Autodesk Inventor part; units mm, degrees
ref_plane "YZ Plane" through (0, 0, 0) normal (1, 0, 0) x (0, 1, 0)
ref_plane "XZ Plane" through (0, 0, 0) normal (0, 1, 0) x (-1, 0, 0)
ref_plane "XY Plane" through (0, 0, 0) normal (0, 0, 1) x (1, 0, 0)
sketch "Sketch6" plane through (0, 0, 0) normal (0, 1, 0) x (-1, 0, 0)
  line L0 (306.3, -490) -> (-306.3, -490)
  line L1 (-306.3, -490) -> (-306.3, 490)
  line L2 (-306.3, 490) -> (306.3, 490)
  line L3 (306.3, 490) -> (306.3, -490)
  line L4 (306.3, -490) -> (-306.3, 490) construction
  line L5 (-306.3, -490) -> (306.3, 490) construction
  point P0 (0, 0)
  dimension "d52" = 612.6
  dimension "d53" = 980
extrude "Plate2" add sketch "Sketch6" along normal blind 0.5
sketch "Sketch11" plane through (-305.8, 0, 490) normal (-1, 0, 0) x (0, -1, 0)
  line L0 (0, -980) -> (0, 0)
  line L1 (0, 0) -> (-10, 0)
  line L2 (-10, 0) -> (-10, -980)
  line L3 (-10, -980) -> (0, -980)
edge flange "Flange2" height 10 angle 90 thickness 0.5 bend radius 0.5 thickness toward (-1, 0, 0) relief tear relief width 0.5 relief depth 0.25 edges at (-306.3, 0.5, 0) wall of the first edge with corners at (-305.8, 0, -490) (-305.8, 0, 490) (-305.8, 10, 490) (-305.8, 10, -490)
bend "Bend3"
corner "Corner3"
sketch "Sketch12" plane through (-306.3, 9.5, 490) normal (0, 1, 0) x (-1, 0, 0)
  line L0 (0, -980) -> (0, 0)
  line L1 (0, 0) -> (-10, 0)
  line L2 (-10, 0) -> (-10, -980)
  line L3 (-10, -980) -> (0, -980)
edge flange "Flange3" height 10 angle 90 thickness 0.5 bend radius 0.5 thickness toward (0, 1, 0) relief tear relief width 0.5 relief depth 0.25 edges at (-305.8, 10, 0) wall of the first edge with corners at (-306.3, 9.5, -490) (-306.3, 9.5, 490) (-296.3, 9.5, 490) (-296.3, 9.5, -490)
bend "Bend4"
corner "Corner4"
sketch "Sketch13" plane through (305.8, 0, -490) normal (1, 0, 0) x (0, 1, 0)
  line L0 (0, 980) -> (0, 0)
  line L1 (0, 0) -> (10, 0)
  line L2 (10, 0) -> (10, 980)
  line L3 (10, 980) -> (0, 980)
edge flange "Flange4" height 10 angle 90 thickness 0.5 bend radius 0.5 thickness toward (1, 0, 0) relief tear relief width 0.5 relief depth 0.25 edges at (306.3, 0.5, 0) wall of the first edge with corners at (305.8, 0, 490) (305.8, 0, -490) (305.8, 10, -490) (305.8, 10, 490)
bend "Bend5"
corner "Corner5"
sketch "Sketch14" plane through (306.3, 9.5, -490) normal (0, 1, 0) x (-1, 0, 0)
  line L0 (0, 980) -> (0, 0)
  line L1 (0, 0) -> (10, 0)
  line L2 (10, 0) -> (10, 980)
  line L3 (10, 980) -> (0, 980)
edge flange "Flange5" height 10 angle 90 thickness 0.5 bend radius 0.5 thickness toward (0, 1, 0) relief tear relief width 0.5 relief depth 0.25 edges at (305.8, 10, 0) wall of the first edge with corners at (306.3, 9.5, 490) (306.3, 9.5, -490) (296.3, 9.5, -490) (296.3, 9.5, 490)
bend "Bend6"
corner "Corner6"
fillet "Corner Round1" radius 4 4 edges at (296.3, 9.75, -490) (296.3, 9.75, 490) (-296.3, 9.75, -490) (-296.3, 9.75, 490)
equation "\"d52\" = ЖАБРЫ_базовая_ширина - 3 * ЖАБРЫ_шаг_листов"
equation "\"d53\" = ЖАБРЫ_базовая_длина_кор_лист"
equation "\"d54\" = Thickness"
equation "\"d84\" = BendReliefWidth"
equation "\"d85\" = BendReliefDepth"
equation "\"d86\" = MinimumRemnant"
equation "\"d87\" = TransitionRadius"
equation "\"d90\" = BendRadius"
equation "\"d91\" = CornerReliefSize"
equation "\"d92\" = GapSize"
equation "\"d93\" = JacobiRadiusSize"
equation "\"d94\" = BendReliefWidth"
equation "\"d95\" = BendReliefDepth"
equation "\"d96\" = MinimumRemnant"
equation "\"d97\" = TransitionRadius"
equation "\"d100\" = BendRadius"
equation "\"d101\" = CornerReliefSize"
equation "\"d102\" = GapSize"
equation "\"d103\" = JacobiRadiusSize"
equation "\"d104\" = BendReliefWidth"
equation "\"d105\" = BendReliefDepth"
equation "\"d106\" = MinimumRemnant"
equation "\"d107\" = TransitionRadius"
equation "\"d110\" = BendRadius"
equation "\"d111\" = CornerReliefSize"
equation "\"d112\" = GapSize"
equation "\"d113\" = JacobiRadiusSize"
equation "\"d114\" = BendReliefWidth"
equation "\"d115\" = BendReliefDepth"
equation "\"d116\" = MinimumRemnant"
equation "\"d117\" = TransitionRadius"
equation "\"d120\" = BendRadius"
equation "\"d121\" = CornerReliefSize"
equation "\"d122\" = GapSize"
equation "\"d123\" = JacobiRadiusSize"
equation "\"BendRadius\" = Thickness"
equation "\"BendReliefWidth\" = Thickness"
equation "\"BendReliefDepth\" = 0.5 * Thickness"
equation "\"CornerReliefSize\" = 4 * Thickness"
equation "\"MinimumRemnant\" = 2 * Thickness"
equation "\"TransitionRadius\" = BendRadius"
equation "\"JacobiRadiusSize\" = BendRadius"
equation "\"GapSize\" = Thickness"
properties part number "MSC 807 SHEET GILLS" material "Stainless Steel"
Geometry: final body of the model. Coordinates: model frame, mm. Give positions to 0.01 mm unless a question says otherwise; leave off trailing zeros. Loops run counter-clockwise (first coordinate to the right, second up) from the corner with the lowest first, then second, coordinate; pieces in that order, holes last. Notation, with made-up numbers: M 70.25,2.25 L 128.25,2.25 A12 ccw 128.25,19.25 Z; hole C 12.25,-15.75 d3. An arc over 180 degrees is marked long. Put each result on its own line as item: value.
1) Cut plane A-A, the plane y = 3. Return the cut outline in (x, z).
Computed values:
outline: M -306.3,-490 L -305.8,-490 L -305.8,490 L -306.3,490 Z; M 305.8,-490 L 306.3,-490 L 306.3,490 L 305.8,490 Z
2) Cut plane C-C, the plane x = 131.5. Return the cut outline in (y, z).
Computed values:
outline: M 0,-490 L 0.5,-490 L 0.5,490 L 0,490 Z
3) Mould query, pull axis X, two halves, no side actions, for faces 1 (the flat face through (4, 0, 7)), 2 (the flat face through (4, 0.5, 7)). Classes: released by +X, released by -X, zero draft, split by the parting line, or undercut.
Computed values:
face 1: zero draft
face 2: undercut
4) Material intervals for L1, parallel to X at y = 2, z = 277; L2, parallel to Y at x = 276.5, z = 430.5, sorted ascending. Write a range as from..to.
Computed values:
L1: x = -306.3..-305.8, 305.8..306.3
L2: y = 0..0.5
5) First-contact query: P1, Ø3, axis at x = -234.5, z = 112, coming from the +Y side; P2, Ø0.6, axis at y = 10, z = 221, coming from the -X side. Flat tips, straight axial feed; report the tip coordinate or a pass-through.
Computed values:
P1: stops at y = 0.5
P2: stops at x = -306.01
6) Cut plane B-B, the plane z = -318.5. Return the cut outline in (x, y), plus the area to 3 significant figures.
Computed values:
outline: M -306.3,1 A1 ccw -305.3,0 L 305.3,0 A1 ccw 306.3,1 L 306.3,9 A1 ccw 305.3,10 L 296.3,10 L 296.3,9.5 L 305.3,9.5 A0.5 cw 305.8,9 L 305.8,1 A0.5 cw 305.3,0.5 L -305.3,0.5 A0.5 cw -305.8,1 L -305.8,9 A0.5 cw -305.3,9.5 L -296.3,9.5 L -296.3,10 L -305.3,10 A1 ccw -306.3,9 Z
area: 325 mm^2
